```python
from build123d import *

# Parameters (mm, degrees)
SALIENTE_EXTRUIR1_DEPTH = 3.1
CORTAR_EXTRUIR1_DEPTH   = 16.5
CROQUIS3_R              = 3.3
SALIENTE_EXTRUIR2_DEPTH = 6.8
CORTAR_EXTRUIR2_DEPTH   = 3.4
CROQUIS5_R              = 2
SALIENTE_EXTRUIR3_DEPTH = 1
CROQUIS6_R              = 0.75
CORTAR_EXTRUIR3_DEPTH   = 10.894132521


with BuildPart() as part:
    # Croquis1 → Saliente-Extruir1 (new body)
    with BuildSketch(Plane(origin=(0, 0, 0), x_dir=(0, 0, -1), z_dir=(1, 0, 0))):
        Polygon((-4.601481645, 0), (-2.300740823, -3.985), (2.300740823, -3.985), (4.601481645, 0), (2.300740823, 3.985), (-2.300740823, 3.985), align=None)
    extrude(amount=-SALIENTE_EXTRUIR1_DEPTH)

    # Croquis2 → Cortar-Extruir1 (cut, symmetric)
    with BuildSketch(Plane.XY):
        Polygon((-3.1, -3.985), (-2.191933202, 3.985), (-3.527931865, 3.985), align=None)
    extrude(amount=CORTAR_EXTRUIR1_DEPTH, both=True, mode=Mode.SUBTRACT)

    # Croquis3 → Saliente-Extruir2 (add)
    with BuildSketch(Plane(origin=(0, 0, 0), x_dir=(0, 0, -1), z_dir=(1, 0, 0))):
        Circle(CROQUIS3_R)
    extrude(amount=-SALIENTE_EXTRUIR2_DEPTH)

    # Croquis4 → Cortar-Extruir2 (cut, symmetric)
    with BuildSketch(Plane.XY):
        Polygon((-6.8, -3.3), (-6.048024985, 3.3), (-6.8, 3.3), align=None)
    extrude(amount=CORTAR_EXTRUIR2_DEPTH, both=True, mode=Mode.SUBTRACT)

    # Croquis5 → Saliente-Extruir3 (add)
    with BuildSketch(Plane(origin=(0, 0, 0), x_dir=(0, 0, -1), z_dir=(1, 0, 0))):
        Circle(CROQUIS5_R)
    extrude(amount=SALIENTE_EXTRUIR3_DEPTH)

    # Croquis6 → Cortar-Extruir3 (cut, through all)
    with BuildSketch(Plane(origin=(1, 0, 0), x_dir=(0, 0, -1), z_dir=(1, 0, 0))):
        Circle(CROQUIS6_R)
    extrude(amount=-CORTAR_EXTRUIR3_DEPTH, mode=Mode.SUBTRACT)


solid = part.part
```
The listing builds one solid part. Answer for the finished solid, in the listing's coordinates (mm). A direction names the side the tool comes from. Coordinates: 2 decimals unless noted, no trailing zeros. Write each loop counter-clockwise with the first axis right and the second up, starting at its lowest first coordinate (ties: lowest second). Pieces come first, ordered by that corner, then holes. Notation, with made-up numbers: (52, 64.5) - (97, 64.5) arc R24 ccw to (97, 75.5) - close; hole circle Ø4 at (-17.75, 82.25). An arc over 180 degrees is marked (long way). Return JSON: item names as keys, results as strings. Group by question number.
Q1. The part is cut by section C-C on y = -2.5. Write down the section's boundary in (x, z).
Q2. The part is cut by section D-D on z = -1.25. Write down the section's boundary in (x, y) (3 decimals), and give its area (3 significant figures).
Q3. Flat-ended cylindrical pins translate along their axes: pin 1 Ø2 at (x, y) = (-5.5, -1) entering from -Z; pin 2 Ø1.4 at (y, z) = (0, 0) entering from +X; pin 3 Ø2 at (x, y) = (-4.5, 3) entering from -Z; pin 4 Ø4 at (y, z) = (0.5, 1.5) entering from -X. Find the tip coordinate at first contact, or state that the pin passes through.
Q4. The part is cut by section A-A on x = -1. Write down the section's boundary in (y, z) (3 decimals).
Q5. Find the intervals of material crossed by line 1 along Z through (x, y) = (-4.5, 0); line 2 along Z through (x, y) = (-3.75, -0.5), in increasing order. Write a range as [from, to].
Q6. Which of the six approach directions +Z, -Z, +X, -X, +Y, -Y give full straight-line access (tool end or side, diameter ignored) to faces 5 (the cylindrical face through (-4.46, 3.27, 0.43)), 6 (the flat face through (-2, -3.985, 0)), 7 (the flat face through (0, 2, -1))?
Q7. For a pull along Z with two mould halves and no side action, classify faces 1 (the cylindrical face through (-2.71, 0.03, 0.75)), 2 (the flat face through (-1.3, 1.96, -3.47)), 3 (the flat face through (-6.346, 0.687, -0.687)), 4 (the cylindrical face through (0.493, -1.952, 0.434)) as +Z half, -Z half, draft (parallel to the pull), parting line (faces both ways), or undercut.
Q8. The part is cut by section B-B on z = 0. Write down the section's boundary in (x, y) (3 decimals).
Evaluation:
{
 "1": {"outline": "(-6.71, -2.15) - (-2.93, -2.15) - (-2.93, -3.16) - (0, -3.16) - (0, 3.16) - (-2.93, 3.16) - (-2.93, 2.15) - (-6.71, 2.15) - close"},
 "2": {"outline": "(-6.772, -3.054) - (-2.994, -3.054) - (-3.1, -3.985) - (0, -3.985) - (0, -1.561) - (1, -1.561) - (1, 1.561) - (0, 1.561) - (0, 3.985) - (-2.192, 3.985) - (-2.298, 3.054) - (-6.076, 3.054) - close", "area": "47.3 mm2"},
 "3": {"pin 1": "stops at z = -3.3", "pin 2": "passes through", "pin 3": "stops at z = -2.62", "pin 4": "stops at x = -6.59"},
 "4": {"outline": "(-3.985, -2.301) - (0, -4.601) - (3.985, -2.301) - (3.985, 2.301) - (0, 4.601) - (-3.985, 2.301) - close; hole circle Ø1.5 at (0, 0)"},
 "5": {"line 1": "z = [-3.3, -0.75], [0.75, 3.3]", "line 2": "z = [-3.26, -0.56], [0.56, 3.26]"},
 "6": {"face 5": "-X", "face 6": "+Z, -Z, +X, -X, -Y", "face 7": "+X"},
 "7": {"face 1": "undercut", "face 2": "-Z half", "face 3": "draft", "face 4": "parting line"},
 "8": {"outline": "(-6.8, -3.3) - (-3.022, -3.3) - (-3.1, -3.985) - (0, -3.985) - (0, -2) - (1, -2) - (1, -0.75) - (-6.509, -0.75) - close; (-6.339, 0.75) - (1, 0.75) - (1, 2) - (0, 2) - (0, 3.985) - (-2.192, 3.985) - (-2.27, 3.3) - (-6.048, 3.3) - close"}
}
